Part model, mm, in its own coordinate system. A direction names the side the tool comes from. Round coordinates to 2 decimals unless told otherwise and drop trailing zeros. Loops run counter-clockwise (first coordinate to the right, second up) from the corner with the lowest first, then second, coordinate; pieces in that order, holes last.
Autodesk Inventor part; units mm, degrees
ref_plane "YZ Plane" through (0, 0, 0) normal (1, 0, 0) x (0, 1, 0)
ref_plane "XZ Plane" through (0, 0, 0) normal (0, 1, 0) x (-1, 0, 0)
ref_plane "XY Plane" through (0, 0, 0) normal (0, 0, 1) x (1, 0, 0)
sketch "Sketch1" plane through (0, 0, 0) normal (0, 0, 1) x (1, 0, 0)
  line L0 (-6.9059, 7.4416) -> (-6.9059, -42.5584)
  line L1 (-6.9059, -42.5584) -> (45.659, -42.5584)
  line L2 (45.659, -42.5584) -> (-4.341, -42.5584)
  line L3 (-6.9059, 7.4416) -> (45.659, 7.4416)
  line L4 (45.659, 7.4416) -> (45.659, -42.5584)
  point P0 (0, 0)
  dimension "d0" = 50
  dimension "d1" = 50
revolve "Revolution1" add sketch "Sketch1" angle 360 about axis through (45.659, 7.4416, 0) along (0, -1, 0)
shell "Shell1" thickness 5 outward yes removed faces 0
sketch "Sketch2" plane through (45.659, 12.4416, 0) normal (0, 1, 0) x (1, 0, 0)
  circle A0 centre (0, 0) radius 49.1631
  point P0 (-45.659, 0)
extrude "Extrusion1" cut sketch "Sketch2" against normal blind 45
equation "\"BendRadius\" = Thickness"
equation "\"BendReliefWidth\" = Thickness"
equation "\"BendReliefDepth\" = 0.5 * Thickness"
equation "\"CornerReliefSize\" = 4 * Thickness"
equation "\"MinimumRemnant\" = 2 * Thickness"
equation "\"TransitionRadius\" = BendRadius"
equation "\"JacobiRadiusSize\" = BendRadius"
equation "\"GapSize\" = Thickness"
properties part number "box" material "Steel, Carbon"
1) Wall check: line 1 along X through (y, z) = (9, 0); line 2 along X through (y, z) = (-19, 0); line 3 along Z through (x, y) = (47, -3). Give the ranges that are in metal, low to high.
Values:
line 1: x = -11.91 to -3.5, 94.82 to 103.22
line 2: x = -11.91 to -6.91, 98.22 to 103.22
line 3: z = -57.55 to -52.55, 52.55 to 57.55
2) Drop flat-ended pins along their axis: pin 1 Ø3 at (y, z) = (-8, 20.5) entering from +X; pin 2 Ø12 at (y, z) = (6, 43.5) entering from -X; pin 3 Ø5 at (y, z) = (-41.5, -32) entering from +X. Give the stop position or say it passes through.
Values:
pin 1: stops at x = 100
pin 2: stops at x = 1.98
pin 3: stops at x = 95.09
3) Slice it at C-C, the plane x = 93. Give the cut face in (y, z).
Values:
outline: (-47.56, -32.75) - (12.44, -32.75) - (12.44, -13.26) - (7.44, -13.26) - (7.44, -22.85) - (-42.56, -22.85) - (-42.56, 22.85) - (7.44, 22.85) - (7.44, 13.26) - (12.44, 13.26) - (12.44, 32.75) - (-47.56, 32.75) - close
4) Mould opens along Y. For faces 1 (the face through (46, -47.558, -1)), 2 (the face through (-2.9, -17.91, 20.13)), 3 (the face through (3, 12.442, -26)) say: released by +Y, released by -Y, zero draft, split by the parting line, or undercut.
Values:
face 1: released by -Y
face 2: undercut
face 3: released by +Y
5) Slice it at B-B, the plane y = -0.5. Give the cut face in (x, z).
Values:
outline: circle Ø115.13 at (45.66, 0); hole circle Ø105.13 at (45.66, 0)
6) Tool access for faces 4 (the face through (58.138, -17.978, 56.196)), 5 (the face through (6.64, 9.98, 29.91)), 6 (the face through (15, 7.442, 39)): list every direction of +Z, -Z, +X, -X, +Y, -Y with a clear straight run to the whole face (end or side of a thin tool).
Values:
face 4: +Y, -Y
face 5: +Y
face 6: none
7) Slice it at A-A, the plane z = 0. Give the cut face in (x, y), then the cut area to 3 significant figures.
Values:
outline: (-11.91, -47.56) - (103.22, -47.56) - (103.22, 12.44) - (94.82, 12.44) - (94.82, 7.44) - (98.22, 7.44) - (98.22, -42.56) - (-6.91, -42.56) - (-6.91, 7.44) - (-3.5, 7.44) - (-3.5, 12.44) - (-11.91, 12.44) - close
area: 1,160 mm2
